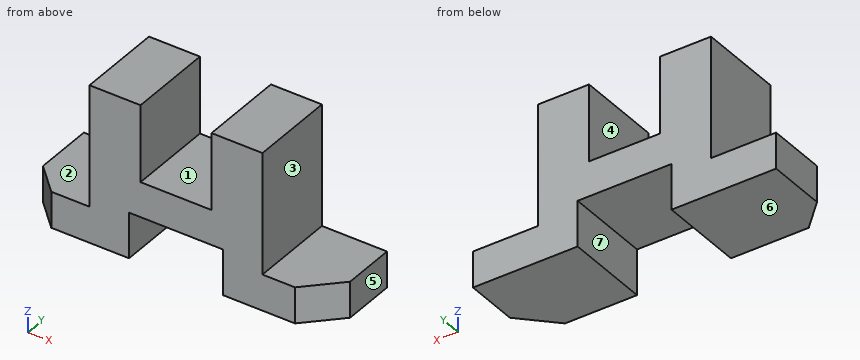
from build123d import *

# Parameters (mm, degrees)
F1_DEPTH = 32
F3_DEPTH = 13.419725
F5_DEPTH = 13.419725


with BuildPart() as f1:
    # F0 (on Front) → F1 (new body)
    with BuildSketch(Plane.XZ):
        Polygon((-56.5, 13.418725), (-56.5, 0), (-17.5, 0), (-17.5, 17), (17.5, 17), (17.5, 0), (56.5, 0), (56.5, 13.418725), (32.225927, 13.418725), (32.225927, 58.61873), (13.225927, 58.61873), (13.225927, 30), (-13.225927, 30), (-13.225927, 58.61873), (-32.225927, 58.61873), (-32.225927, 13.418725), align=None)
    extrude(amount=F1_DEPTH)

    # F2 (on face) → F3 (cut, through all)
    with BuildSketch(Plane.XY.offset(13.418725)):
        Polygon((-56.5, -32), (-46.5, -32), (-56.5, -22), align=None)
    extrude(amount=-F3_DEPTH, mode=Mode.SUBTRACT)

    # F4 (on face) → F5 (cut, through all)
    with BuildSketch(Plane.XY.offset(13.418725)):
        Polygon((56.5, -19.862964), (44.362964, -32), (56.5, -32), align=None)
    extrude(amount=-F5_DEPTH, mode=Mode.SUBTRACT)


solid = f1.part
Design review of the part built by this model. Coordinates are the model's own, in mm. Face numbers are marked on the shaded views. A direction names the side the tool comes from. Round coordinates to 2 decimals unless told otherwise and drop trailing zeros. Write each loop counter-clockwise with the first axis right and the second up, starting at its lowest first coordinate (ties: lowest second). Pieces come first, ordered by that corner, then holes. Notation, with made-up numbers: (-28.75, 34) -> (-12.75, 34) arc R17 cw to (-12.75, 66) -> close; hole circle Ø4 at (-37, 84). An arc over 180 degrees is marked (long way). One line per item, written item: value. Start each with the question number.
Q1. Insertion check: P1, Ø12, axis at y = -5.5, z = 32.5, coming from the +X side; P2, Ø3, axis at x = 10.5, y = -16, coming from the +Z side; P3, Ø7.5, axis at x = -42.5, y = -23.5, coming from the +Z side. Each pin has a flat end and moves straight along its axis. Give the tip position at first contact, or say it passes through.
Q2. Add section A-A (z = 7.5). Give the boundary of the cut face in (x, y).
Q3. The part is to be moulded in two halves that separate along X. For the marked faces 4, 5, 6 and 7, say which applies: pulls with the +X half, pulls with the -X half, needs draft (parallel to the pull), parting line crosses it, or undercut.
Q4. To check wall thickness, follow probe 1 along X at (y, z) = (-19.5, 10); probe 2 along X at (y, z) = (-22.5, 36); probe 3 along X at (y, z) = (-30, 18). State the ranges of each line that lie inside material, in increasing order.
Q5. Tool access review of the marked faces 1, 2 and 3: name each direction out of +Z, -Z, +X, -X, +Y, -Y from which nothing blocks a thin tool from reaching the whole face with its end or side.
Q6. Add section C-C (z = 52.5). Give the boundary of the cut face in (x, y), then the cut area to 3 significant figures.
Q7. Add section B-B (y = -7). Give the boundary of the cut face in (x, z).
Q8. Add section D-D (x = -14.5). Give the boundary of the cut face in (y, z), then the cut area to 3 significant figures.
Response:
1. P1: stops at x = 32.23
1. P2: stops at z = 30
1. P3: stops at z = 13.42
2. outline: (-56.5, -22) -> (-46.5, -32) -> (-17.5, -32) -> (-17.5, 0) -> (-56.5, 0) -> close; (17.5, -32) -> (44.36, -32) -> (56.5, -19.86) -> (56.5, 0) -> (17.5, 0) -> close
3. face 4: undercut
3. face 5: pulls with the +X half
3. face 6: needs draft
3. face 7: undercut
4. probe 1: x = -56.5 to -17.5, 17.5 to 56.5
4. probe 2: x = -32.23 to -13.23, 13.23 to 32.23
4. probe 3: x = -32.23 to 32.23
5. face 1: +Z, +Y, -Y
5. face 2: +Z, -X, +Y, -Y
5. face 3: +Z, +X, +Y, -Y
6. outline: (-32.23, -32) -> (-13.23, -32) -> (-13.23, 0) -> (-32.23, 0) -> close; (13.23, -32) -> (32.23, -32) -> (32.23, 0) -> (13.23, 0) -> close
6. area: 1,220 mm^2
7. outline: (-56.5, 0) -> (-17.5, 0) -> (-17.5, 17) -> (17.5, 17) -> (17.5, 0) -> (56.5, 0) -> (56.5, 13.42) -> (32.23, 13.42) -> (32.23, 58.62) -> (13.23, 58.62) -> (13.23, 30) -> (-13.23, 30) -> (-13.23, 58.62) -> (-32.23, 58.62) -> (-32.23, 13.42) -> (-56.5, 13.42) -> close
8. outline: (-32, 17) -> (0, 17) -> (0, 58.62) -> (-32, 58.62) -> close
8. area: 1,330 mm^2
